from build123d import *

# Parameters (mm, degrees)
BOSS_EXTRUDE1_DEPTH = 15
FILLET1_RADIUS      = 7.5
FILLET1_LENGTH      = 1.8
FILLET2_RADIUS      = 7.5
FILLET2_LENGTH      = 1.8
SKETCH3_R           = 2.5
CUT_EXTRUDE1_DEPTH  = 10
SKETCH2_R           = 2.5
CUT_EXTRUDE2_DEPTH  = 10
CHAMFER1_SIZE       = 0.5


with BuildPart() as part:
    # Sketch1 → Boss-Extrude1 (new body)
    with BuildSketch(Plane.XY):
        Polygon((0, 0), (20, 0), (20, 1.8), (1.8, 1.8), (1.8, 20), (0, 20), align=None)
    extrude(amount=BOSS_EXTRUDE1_DEPTH)

    # Fillet1: full round fillet: the end face becomes a half cylinder, R = half its width
    fillet1_face = Plane((0.9, 20, 7.5), x_dir=(1, 0, 0), z_dir=(0, 1, 0))  # on the end face: x along it, z out of the body
    fillet1_slab = fillet1_face.offset(-FILLET1_RADIUS / 2) * Box(FILLET1_LENGTH, 2 * FILLET1_RADIUS, FILLET1_RADIUS, mode=Mode.PRIVATE)  # the body's end, R deep
    fillet1_round = Plane((0.9, 12.5, 7.5), x_dir=(0, 1, 0), z_dir=(1, 0, 0)) * Cylinder(FILLET1_RADIUS, FILLET1_LENGTH, mode=Mode.PRIVATE)  # its axis R under the face
    add(fillet1_slab - fillet1_round, mode=Mode.SUBTRACT)

    # Fillet2: full round fillet: the end face becomes a half cylinder, R = half its width
    fillet2_face = Plane((20, 0.9, 7.5), x_dir=(0, -1, 0), z_dir=(1, 0, 0))  # on the end face: x along it, z out of the body
    fillet2_slab = fillet2_face.offset(-FILLET2_RADIUS / 2) * Box(FILLET2_LENGTH, 2 * FILLET2_RADIUS, FILLET2_RADIUS, mode=Mode.PRIVATE)  # the body's end, R deep
    fillet2_round = Plane((12.5, 0.9, 7.5), x_dir=(1, 0, 0), z_dir=(0, -1, 0)) * Cylinder(FILLET2_RADIUS, FILLET2_LENGTH, mode=Mode.PRIVATE)  # its axis R under the face
    add(fillet2_slab - fillet2_round, mode=Mode.SUBTRACT)

    # Sketch3 → Cut-Extrude1 (cut)
    with BuildSketch(Plane(origin=(0, 1.8, 0), x_dir=(1, 0, 0), z_dir=(0, 1, 0))):
        with Locations(Location((11.8, -7.5, 0), (0, 0, 180))):
            Circle(SKETCH3_R)
    extrude(amount=-CUT_EXTRUDE1_DEPTH, mode=Mode.SUBTRACT)

    # Sketch2 → Cut-Extrude2 (cut)
    with BuildSketch(Plane(origin=(1.8, 0, 0), x_dir=(0, 0, -1), z_dir=(1, 0, 0))):
        with Locations((-7.5, 11.8)):
            Circle(SKETCH2_R)
    extrude(amount=-CUT_EXTRUDE2_DEPTH, mode=Mode.SUBTRACT)

    # Chamfer1
    chamfer1_edges = [part.edges().sort_by_distance(p)[0] for p in [
        (14.3, 0, 7.5),
        (14.3, 1.8, 7.5),
        (0, 11.8, 10),
        (1.8, 11.8, 10),
    ]]
    chamfer(chamfer1_edges, length=CHAMFER1_SIZE)


solid = part.part
Could you check a few things on this model? Use its own coordinates, in mm. A direction names the side the tool comes from. Give positions to 0.01 mm unless a question says otherwise; leave off trailing zeros. Order: outer loops, then holes, each group sorted by start corner. A loop starts at its lowest first (then second) coordinate and runs counter-clockwise, first axis right, second up. Notation, with made-up numbers: (-19.75, 37) - (24.25, 37) arc R32 ccw to (24.25, 71) - close; hole circle Ø1 at (16.5, 33.5). An arc over 180 degrees is marked (long way). Return JSON: item names as keys, results as strings. Group by question number.
Q1. Thinking about a two-plate mould opening in Z: for faces 3 (the face through (1.6, 4, 0)), 4 (the face through (0.91, 14.28, 7.83)), 5 (the face through (1.6, 4, 15)), which applies, pulls with the +Z half, pulls with the -Z half, needs draft (parallel to the pull), parting line crosses it, or undercut?
Q2. Please list where these lines run through material, in increasing order: line 1 along Y through (x, z) = (1, 7.5); line 2 along X through (y, z) = (16, 13.75); line 3 along Y through (x, z) = (1, 7). Write a range as [from, to].
Q3. Suppose I cut it at D-D, the plane z = 12. Please give me the cut outline in (x, y), and give its area (3 significant figures).
Q4. Will these pins go through, and if not, where does the flat tip stop? pin 1 Ø3 at (y, z) = (16.5, 5) entering from +X; pin 2 Ø1.5 at (x, z) = (15, 2) entering from +Y.
Q5. Which directions (+Z, -Z, +X, -X, +Y, -Y) give clear straight access to the entire face, cutting with the end or side of a thin tool? Please do faces 1 (the face through (9, 1.8, 9)), 2 (the face through (20, 0.89, 7.34)).
Q6. Suppose I cut it at A-A, the plane y = 11.8. Please give me the cut outline in (x, z), and give its area (3 significant figures).
Q7. Suppose I cut it at B-B, the plane z = 7.5. Please give me the cut outline in (x, y).
Resolved:
{
 "1": {"face 3": "pulls with the -Z half", "face 4": "undercut", "face 5": "pulls with the +Z half"},
 "2": {"line 1": "y = [0, 9.3], [14.3, 20]", "line 2": "x = [0, 1.8]", "line 3": "y = [0, 9.35], [14.25, 19.98]"},
 "3": {"outline": "(0, 0) - (18.5, 0) - (18.5, 1.8) - (1.8, 1.8) - (1.8, 18.5) - (0, 18.5) - close", "area": "63.4 mm2"},
 "4": {"pin 1": "stops at x = 1.8", "pin 2": "stops at y = 1.8"},
 "5": {"face 1": "+Z, -Z, +X, +Y", "face 2": "+X, +Y, -Y"},
 "6": {"outline": "(0, 0) - (1.8, 0) - (1.8, 4.5) - (1.3, 5) - (0.5, 5) - (0, 4.5) - close; (0, 10.5) - (0.5, 10) - (1.3, 10) - (1.8, 10.5) - (1.8, 15) - (0, 15) - close", "area": "17.5 mm2"},
 "7": {"outline": "(0, 0) - (8.8, 0) - (9.3, 0.5) - (9.3, 1.3) - (8.8, 1.8) - (1.8, 1.8) - (1.8, 8.8) - (1.3, 9.3) - (0.5, 9.3) - (0, 8.8) - close; (0, 14.8) - (0.5, 14.3) - (1.3, 14.3) - (1.8, 14.8) - (1.8, 20) - (0, 20) - close; (14.3, 0.5) - (14.8, 0) - (20, 0) - (20, 1.8) - (14.8, 1.8) - (14.3, 1.3) - close"}
}
